from build123d import *

# Parameters (mm, degrees)
F0_W     = 98.5
F0_H     = 38
F1_DEPTH = 2
F3_DEPTH = 35
F4_W     = 9
F4_H     = 9.55
F5_DEPTH = 3
F6_R     = 1.5
F7_DEPTH = 1.5
F8_R     = 0.74999


# Not quite as in the source:
# - a fillet or chamfer is up to 0.001 mm smaller than in the source, because OpenCascade refuses the exact size


with BuildPart() as f1:
    # F0 (on Top) → F1 (new body)
    with BuildSketch(Plane.XY):
        with Locations((49.25, 19)):
            Rectangle(F0_W, F0_H)
    extrude(amount=F1_DEPTH)

    # F2 (on face) → F3 (join)
    with BuildSketch(Plane(origin=(0, 38, 0), x_dir=(-1, 0, 0), z_dir=(0, 1, 0))):
        Polygon((-101, 0), (-98.5, 0), (-98.5, 7), (-92, 7), (-92, 9.55), (-101, 9.55), align=None)
        Polygon((0, 7), (0, 0), (2.5, 0), (2.5, 9.55), (-6.5, 9.55), (-6.5, 7), align=None)
    extrude(amount=-F3_DEPTH)

    # F4 (on face) → F5 (join)
    with BuildSketch(Plane.XZ.offset(-3)):
        with Locations((2, 4.775)):
            Rectangle(F4_W, F4_H)
        with Locations((96.5, 4.775)):
            Rectangle(F4_W, F4_H)
    extrude(amount=F5_DEPTH)

    # F6 (on face) → F7 (join)
    with BuildSketch(Plane.YZ):
        with Locations((6.5, 4.25)):
            Circle(F6_R)
    extrude(amount=F7_DEPTH)

    # F8 (radius 0.75 in the source; OpenCascade refuses exactly that, so slightly less here)
    f8_edges = [f1.edges().sort_by_distance(p)[0] for p in [
        (1.5, 5, 4.25),
        (0, 5, 4.25),
    ]]
    fillet(f8_edges, radius=F8_R)


solid = f1.part
The model under review builds one solid part; all positions refer to its coordinate system, in mm. A direction names the side the tool comes from. Round coordinates to 2 decimals unless told otherwise and drop trailing zeros. Loops run counter-clockwise (first coordinate to the right, second up) from the corner with the lowest first, then second, coordinate; pieces in that order, holes last. Notation, with made-up numbers: (-25.5, 21) -> (0.5, 21) arc R32 cw to (0.5, 48) -> close; hole circle Ø10 at (8, 16.25). An arc over 180 degrees is marked (long way). Return JSON: item names as keys, results as strings.
(1) Add section A-A on z = 8.25. Write out the cut boundary in (x, y), plus the area to 3 significant figures.
Solved:
{"outline": "(-2.5, 0) -> (6.5, 0) -> (6.5, 38) -> (-2.5, 38) -> close; (92, 0) -> (101, 0) -> (101, 38) -> (92, 38) -> close", "area": "684 mm2"}
(2) For pin 1 (1.5 mm diameter, centred on x = 3, z = 5.5, fed in from +Y); pin 2 (12 mm diameter, centred on x = 78, y = 5, fed in from +Z), all flat-tipped, find the tip position at first contact; note any pin that passes through.
Solved:
{"pin 1": "y = 3", "pin 2": "z = 2"}
(3) Add section C-C on x = 10.5. Write out the cut boundary in (y, z).
Solved:
{"outline": "(0, 0) -> (38, 0) -> (38, 2) -> (0, 2) -> close"}
(4) The part is to be moulded in two halves that separate along X. For faces 5 (the flat face through (98.5, 21, 4)), 6 (the flat face through (101, 19, 5)), 7 (the flat face through (49, 38, 1)), 8 (the flat face through (-2.5, 19, 5)), say which applies: released by +X, released by -X, zero draft, split by the parting line, or undercut.
Solved:
{"face 5": "undercut", "face 6": "released by +X", "face 7": "zero draft", "face 8": "released by -X"}
(5) For line 1 (X direction, y = 31, z = 3.25); line 2 (X direction, y = 6.5, z = 8); line 3 (Z direction, x = 2.5, y = 26), list the stretches that pass through material, from the lowest coordinate up.
Solved:
{"line 1": "-2.5 to 0, 98.5 to 101", "line 2": "-2.5 to 6.5, 92 to 101", "line 3": "0 to 2, 7 to 9.55"}
(6) For faces 1 (the flat face through (95, 3, 5)), 2 (the flat face through (92, 15, 7.4)), 3 (the flat face through (3, 3, 5)), 4 (the flat face through (2, 19, 9.55)), list the 3-axis set-ups (+Z, -Z, +X, -X, +Y, -Y) from which the entire face can be reached by the end or side of a thin tool; tool diameter is ignored.
Solved:
{"face 1": "+Y", "face 2": "+Z, +Y, -Y", "face 3": "none", "face 4": "+Z, +X, -X, +Y, -Y"}
(7) Add section B-B on y = 19. Write out the cut boundary in (x, z).
Solved:
{"outline": "(-2.5, 0) -> (101, 0) -> (101, 9.55) -> (92, 9.55) -> (92, 7) -> (98.5, 7) -> (98.5, 2) -> (0, 2) -> (0, 7) -> (6.5, 7) -> (6.5, 9.55) -> (-2.5, 9.55) -> close"}
